The model under review builds one solid part; all positions refer to its coordinate system, in mm. A direction names the side the tool comes from. Round coordinates to 2 decimals unless told otherwise and drop trailing zeros. Loops run counter-clockwise (first coordinate to the right, second up) from the corner with the lowest first, then second, coordinate; pieces in that order, holes last. Notation, with made-up numbers: M 32,80 L 40,80 A21 cw 40,94 Z; hole C 82,-24 d7. An arc over 180 degrees is marked long. Answer in a Markdown table with one row per item. Add a question column.
from build123d import *

# Parameters (mm, degrees)
ESBO_O1_W              = 42.3
ESBO_O1_H              = 42.3
UPPERBODY_DEPTH        = 8
CHANFRO1_SIZE          = 4
ESBO_O2_R              = 11
ESBO_O2_R_2            = 4.1
LITTLETOPCIRCLE_DEPTH  = 1.5
ESBO_O3_R              = 1.853680608
MOUNTINGHOLES_DEPTH    = 25
PADR_OCIRCULAR1_COUNT  = 4
LITTLEMETALTABS_DEPTH  = 3
PADR_OCIRCULAR2_COUNT  = 4
MIDDLEBODY_DEPTH       = 22
FILETE1_R              = 6
ESBO_O9_W              = 42.3
ESBO_O9_H              = 42.3
BOTTOMBODY_DEPTH       = 8
CHANFRO5_SIZE          = 4
LITTLEMETALTABS2_DEPTH = 3
PADR_OCIRCULAR3_COUNT  = 4
ESBO_O4_R              = 4
BOSS_EXTRUDE1_DEPTH    = 25.4


with BuildPart() as part:
    # Esbo_o1 → UpperBody (new body)
    with BuildSketch(Plane(origin=(0, 0, 0), x_dir=(1, 0, 0), z_dir=(0, 1, 0))):
        Rectangle(ESBO_O1_W, ESBO_O1_H)
    extrude(amount=UPPERBODY_DEPTH)

    # Chanfro1
    chanfro1_edges = [part.edges().sort_by_distance(p)[0] for p in [
        (21.15, 4, 21.15),
        (-21.15, 4, 21.15),
        (-21.15, 4, -21.15),
        (21.15, 4, -21.15),
    ]]
    chamfer(chanfro1_edges, length=CHANFRO1_SIZE)

    # Esbo_o2 → LittleTopCircle (add)
    with BuildSketch(Plane(origin=(0, 8, 0), x_dir=(1, 0, 0), z_dir=(0, 1, 0))):
        Circle(ESBO_O2_R)
        Circle(ESBO_O2_R_2, mode=Mode.SUBTRACT)
    extrude(amount=LITTLETOPCIRCLE_DEPTH)

    # Esbo_o3 → MountingHoles (cut)
    with BuildSketch(Plane(origin=(0, 8, 0), x_dir=(1, 0, 0), z_dir=(0, 1, 0))):
        with Locations((-15.5, 15.5)):
            Circle(ESBO_O3_R)
    mountingholes = extrude(amount=-MOUNTINGHOLES_DEPTH, mode=Mode.SUBTRACT)

    # Padr_oCircular1: MountingHoles ×4 about axis
    padr_ocircular1_axis = Axis((0, 0, 0), (0, 1, 0))
    for i in range(1, PADR_OCIRCULAR1_COUNT):
        add(mountingholes.rotate(padr_ocircular1_axis, i * 360 / PADR_OCIRCULAR1_COUNT), mode=Mode.SUBTRACT)

    # Esbo_o7 → LittleMetalTabs (add)
    with BuildSketch(Plane.XZ):
        Polygon((-19.65, -16.528679656), (-21.15, -16.528679656), (-21.15, -17.15), (-17.15, -21.15), (-16.528679656, -21.15), (-16.528679656, -19.65), align=None)
    littlemetaltabs = extrude(amount=LITTLEMETALTABS_DEPTH)

    # Padr_oCircular2: LittleMetalTabs ×4 about axis
    padr_ocircular2_axis = Axis((0, 0, 0), (0, 1, 0))
    for i in range(1, PADR_OCIRCULAR2_COUNT):
        add(littlemetaltabs.rotate(padr_ocircular2_axis, i * 360 / PADR_OCIRCULAR2_COUNT))

    # Esbo_o8 → MiddleBody (add)
    with BuildSketch(Plane.XZ):
        Polygon((-14.9, 21.1), (14.9, 21.1), (21.1, 14.9), (21.1, -14.9), (14.9, -21.1), (-14.9, -21.1), (-21.1, -14.9), (-21.1, 14.9), align=None)
    extrude(amount=MIDDLEBODY_DEPTH)

    # Filete1
    filete1_edges = [part.edges().sort_by_distance(p)[0] for p in [
        (-21.1, -11, -14.9),
        (-14.9, -11, -21.1),
        (14.9, -11, -21.1),
        (21.1, -11, -14.9),
        (21.1, -11, 14.9),
        (14.9, -11, 21.1),
        (-14.9, -11, 21.1),
        (-21.1, -11, 14.9),
    ]]
    fillet(filete1_edges, radius=FILETE1_R)

    # Esbo_o9 → BottomBody (add)
    with BuildSketch(Plane.XZ.offset(22)):
        Rectangle(ESBO_O9_W, ESBO_O9_H)
    extrude(amount=BOTTOMBODY_DEPTH)

    # Chanfro5
    chanfro5_edges = [part.edges().sort_by_distance(p)[0] for p in [
        (21.15, -26, -21.15),
        (21.15, -26, 21.15),
        (-21.15, -26, 21.15),
        (-21.15, -26, -21.15),
    ]]
    chamfer(chanfro5_edges, length=CHANFRO5_SIZE)

    # Esbo_o10 → LittleMetalTabs2 (add)
    with BuildSketch(Plane(origin=(0, -22, 0), x_dir=(1, 0, 0), z_dir=(0, 1, 0))):
        Polygon((-16.528679656, -21.15), (-16.528679656, -19.65), (-19.65, -16.528679656), (-21.15, -16.528679656), (-21.15, -17.15), (-17.15, -21.15), align=None)
    littlemetaltabs2 = extrude(amount=LITTLEMETALTABS2_DEPTH)

    # Padr_oCircular3: LittleMetalTabs2 ×4 about axis
    padr_ocircular3_axis = Axis((0, 0, 0), (0, 1, 0))
    for i in range(1, PADR_OCIRCULAR3_COUNT):
        add(littlemetaltabs2.rotate(padr_ocircular3_axis, i * 360 / PADR_OCIRCULAR3_COUNT))

    # Esbo_o4 → Boss-Extrude1 (add)
    with BuildSketch(Plane(origin=(0, 8, 0), x_dir=(1, 0, 0), z_dir=(0, 1, 0))):
        Circle(ESBO_O4_R)
    extrude(amount=BOSS_EXTRUDE1_DEPTH)


solid = part.part
1. Take a section at B-B, the plane x = 0. State the section outline as (y, z) points, and give its area (3 significant figures).
2. To check wall thickness, follow probe 1 along Z at (x, y) = (-15.5, 5.5). State the ranges of the line that lie inside material, in increasing order.
3. Take a section at A-A, the plane y = 2.5. State the section outline as (x, z) points.
4. Mouldability with a two-part tool opening along X and no side actions: class faces 6 (the flat face through (-20.5, -22, 15.8)), 7 (the flat face through (-20, -21, 16.529)), 8 (the flat face through (-19.1, 2.6, 19.2)) as released by +X, released by -X, zero draft, split by the parting line, or undercut.
5. Take a section at C-C, the plane z = 0. State the section outline as (x, y) points.
6. For pin 1 Ø17.5 at (y, z) = (-13.5, -1) entering from +X; pin 2 Ø1.6 at (y, z) = (-20.5, 20.5) entering from -X; pin 3 Ø5 at (x, z) = (-18, -19.5) entering from +Y; pin 4 Ø1.6 at (y, z) = (-1.5, 20.5) entering from +X, all flat-tipped, find the tip position at first contact; note any pin that passes through.
7. Machinability: for faces 1 (the flat face through (16.529, -21, -20)), 2 (the flat face through (-20.5, 0, -15.8)), 3 (the flat face through (-15, 0, -15)), 4 (the flat face through (-19, -3, 19)), 5 (the flat face through (19, -3, -19)), which of the approach directions +Z, -Z, +X, -X, +Y, -Y give a long, thin tool a straight path to every point of the face, cutting with its end or side? Answer none if there is none.
8. Take a section at D-D, the plane y = 15. State the section outline as (x, z) points, and give its area (3 significant figures).
Check sheet entries:
| question | item | result |
|---|---|---|
| 1 | outline | M -30,-21.15 L -22,-21.15 L -22,-21.1 L 0,-21.1 L 0,-21.15 L 8,-21.15 L 8,-11 L 9.5,-11 L 9.5,-4.1 L 8,-4.1 L 8,-4 L 33.4,-4 L 33.4,4 L 8,4 L 8,4.1 L 9.5,4.1 L 9.5,11 L 8,11 L 8,21.15 L 0,21.15 L 0,21.1 L -22,21.1 L -22,21.15 L -30,21.15 Z |
| 1 | area | 1,830 mm^2 |
| 2 | probe 1 | z = -21.15 to -17.35, -13.65 to 13.65, 17.35 to 21.15 |
| 3 | outline | M -21.15,-17.15 L -17.15,-21.15 L 17.15,-21.15 L 21.15,-17.15 L 21.15,17.15 L 17.15,21.15 L -17.15,21.15 L -21.15,17.15 Z; hole C -15.5,-15.5 d3.71; hole C -15.5,15.5 d3.71; hole C 15.5,-15.5 d3.71; hole C 15.5,15.5 d3.71 |
| 4 | face 6 | undercut |
| 4 | face 7 | zero draft |
| 4 | face 8 | released by -X |
| 5 | outline | M -21.15,-30 L 21.15,-30 L 21.15,-22 L 21.1,-22 L 21.1,0 L 21.15,0 L 21.15,8 L 11,8 L 11,9.5 L 4.1,9.5 L 4.1,8 L 4,8 L 4,33.4 L -4,33.4 L -4,8 L -4.1,8 L -4.1,9.5 L -11,9.5 L -11,8 L -21.15,8 L -21.15,0 L -21.1,0 L -21.1,-22 L -21.15,-22 Z |
| 6 | pin 1 | stops at x = 21.15 |
| 6 | pin 2 | stops at x = -18.6 |
| 6 | pin 3 | stops at y = 8 |
| 6 | pin 4 | stops at x = 18.6 |
| 7 | face 1 | -Z |
| 7 | face 2 | none |
| 7 | face 3 | +Y |
| 7 | face 4 | +Z, -X |
| 7 | face 5 | -Z, +X |
| 8 | outline | C 0,0 d8 |
| 8 | area | 50.3 mm^2 |
